Geometry: final body of the model. Coordinates: model frame, mm. Coordinates: 2 decimals unless noted, no trailing zeros. Loops run counter-clockwise (first coordinate to the right, second up) from the corner with the lowest first, then second, coordinate; pieces in that order, holes last. Notation, with made-up numbers: (-38.5, 76.5) - (-26.5, 76.5) arc R21 ccw to (-26.5, 107.5) - close; hole circle Ø3 at (35, 56.25). An arc over 180 degrees is marked (long way). Return JSON: item names as keys, results as strings.
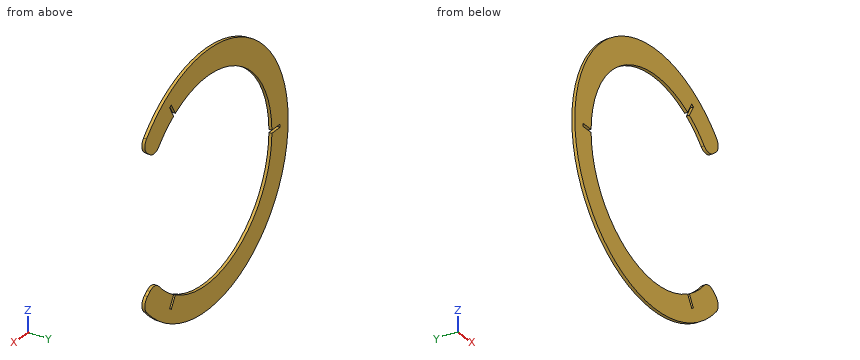
from build123d import *

# Parameters (mm, degrees)
SKETCH1_R           = 125
BOSS_EXTRUDE1_DEPTH = 3
SKETCH2_R           = 100
CUT_EXTRUDE1_DEPTH  = 3
SKETCH3_W           = 25
SKETCH3_H           = 3
CUT_EXTRUDE2_DEPTH  = 3
CIRPATTERN1_COUNT   = 3
CUT_EXTRUDE3_DEPTH  = 3
FILLET1_R           = 10


with BuildPart() as part:
    # Sketch1 → Boss-Extrude1 (new body)
    with BuildSketch(Plane(origin=(0, 0, 0), x_dir=(1, 0, 0), z_dir=(0, 1, 0))):
        with Locations(Location((0, 0, 0), (0, 0, 270))):
            Circle(SKETCH1_R)
    extrude(amount=BOSS_EXTRUDE1_DEPTH)

    # Sketch2 → Cut-Extrude1 (cut)
    with BuildSketch(Plane(origin=(0, 3, 0), x_dir=(1, 0, 0), z_dir=(0, 1, 0))):
        with Locations(Location((0, 0, 0), (0, 0, 270))):
            Circle(SKETCH2_R)
    extrude(amount=-CUT_EXTRUDE1_DEPTH, mode=Mode.SUBTRACT)

    # Sketch3 → Cut-Extrude2 (cut)
    with BuildSketch(Plane(origin=(0, 3, 0), x_dir=(1, 0, 0), z_dir=(0, 1, 0))):
        with Locations((-100, 0)):
            Rectangle(SKETCH3_W, SKETCH3_H)
    cut_extrude2 = extrude(amount=-CUT_EXTRUDE2_DEPTH, mode=Mode.SUBTRACT)

    # CirPattern1: Cut-Extrude2 ×3 about axis
    cirpattern1_axis = Axis((0, 0, 0), (0, 1, 0))
    for i in range(1, CIRPATTERN1_COUNT):
        add(cut_extrude2.rotate(cirpattern1_axis, i * 360 / CIRPATTERN1_COUNT), mode=Mode.SUBTRACT)

    # Sketch4 → Cut-Extrude3 (cut)
    with BuildSketch(Plane(origin=(0, 3, 0), x_dir=(1, 0, 0), z_dir=(0, 1, 0))):
        with BuildLine():
            Line((80, -60), (99.982550279, -75.023260657))
            ThreePointArc((99.982550279, -75.023260657), (124.999999154, -0.014539179), (100, 75))
            Line((100, 75), (80, 60))
            ThreePointArc((80, 60), (100, 0), (80, -60))
        make_face()
    extrude(amount=-CUT_EXTRUDE3_DEPTH, mode=Mode.SUBTRACT)

    # Fillet1
    fillet1_edges = [part.edges().sort_by_distance(p)[0] for p in [
        (80, 1.5, 60),
        (80, 1.5, -60),
        (100, 1.5, -75),
        (99.982550279, 1.5, 75.023260657),
    ]]
    fillet(fillet1_edges, radius=FILLET1_R)


solid = part.part
Item 1: First-contact query: pin 1 Ø0.9 at (x, y) = (-104.5, 1) entering from +Z; pin 2 Ø1.5 at (y, z) = (1, 0.5) entering from +X. Flat tips, straight axial feed; report the tip coordinate or a pass-through.
Worked out:
{"pin 1": "z = 69.27", "pin 2": "x = -112.5"}
Item 2: Ray query, probe 1 along Z at (x, y) = (-59.5, 2.35); probe 2 along Z at (x, y) = (32, 0.45); probe 3 along X at (y, z) = (0.95, 3). Return the intervals inside material, ascending. Write a range as from..to.
Worked out:
{"probe 1": "-109.93..-80.37, 80.37..109.93", "probe 2": "-120.83..-94.74, 94.74..120.83", "probe 3": "-124.96..-99.95"}
Item 3: Section query C-C, the plane x = -68. Return loops of the section in (y, z).
Worked out:
{"outline": "(0, -104.89) - (3, -104.89) - (3, -73.32) - (0, -73.32) - close; (0, 73.32) - (3, 73.32) - (3, 104.89) - (0, 104.89) - close"}
Item 4: Section query B-B, the plane y = 1.5. Return loops of the section in (x, z), and give its area (3 significant figures).
Worked out:
{"outline": "(-112.5, -1.5) - (-112.5, 1.5) - (-99.99, 1.5) arc R100 cw to (48.7, 87.34) - (54.95, 98.18) - (57.55, 96.68) - (51.29, 85.84) arc R100 cw to (74.21, 67.03) arc R10 ccw to (87.64, 65.74) - (91.65, 68.76) arc R10 ccw to (93.09, 83.43) arc R125 ccw (long way) to (93.1, -83.41) arc R10 ccw to (91.65, -68.74) - (87.64, -65.73) arc R10 ccw to (74.21, -67.02) arc R100 cw to (51.29, -85.84) - (57.55, -96.68) - (54.95, -98.18) - (48.7, -87.34) arc R100 cw to (-99.99, -1.5) - close", "area": "13,900 mm^2"}
Item 5: Section query D-D, the plane z = 52. Return loops of the section in (x, y), and give its area (3 significant figures).
Worked out:
{"outline": "(-113.67, 0) - (-85.42, 0) - (-85.42, 3) - (-113.67, 3) - close", "area": "84.8 mm^2"}
Item 6: Section query A-A, the plane x = 0. Return loops of the section in (y, z), and give its area (3 significant figures).
Worked out:
{"outline": "(0, -125) - (3, -125) - (3, -100) - (0, -100) - close; (0, 100) - (3, 100) - (3, 125) - (0, 125) - close", "area": "150 mm^2"}
